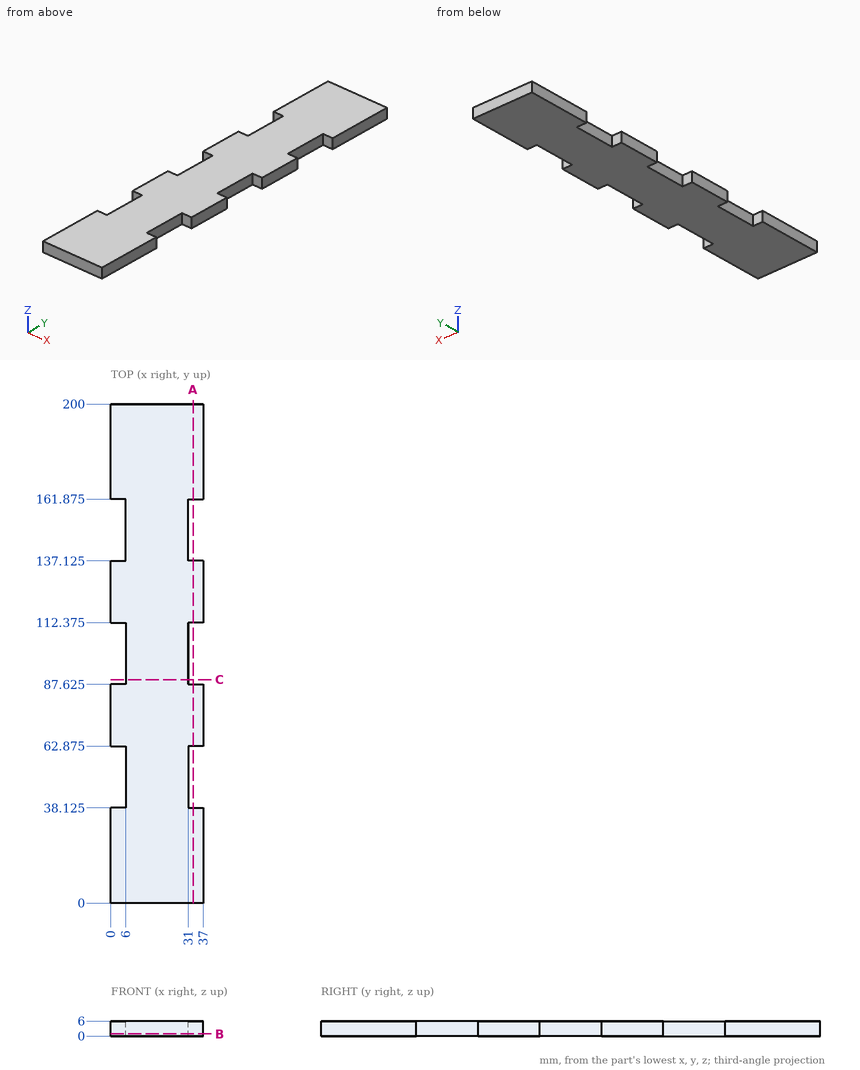
Answer from the drawing. Dimensions are ordinates in mm from the lowest x, y and z of the part. Round coordinates to 2 decimals unless told otherwise and drop trailing zeros. Loops run counter-clockwise (first coordinate to the right, second up) from the corner with the lowest first, then second, coordinate; pieces in that order, holes last.
Q1. Section C-C on y = 89.5 is taken. Write down the section's boundary in (x, z).
Q2. Each of these flat-tipped pins is pushed along its axis until it touches: pin 1 (3 mm diameter, centred on y = 148.5, z = 3, fed in from +X); pin 2 (1 mm diameter, centred on y = 49, z = 3, fed in from -X). Where does it stop, or does it pass through?
Q3. Section B-B on z = 0.9 is taken. Write down the section's boundary in (x, y) (3 decimals), and give its area (3 significant figures).
Q4. Consider probe 1 along Y at (x, z) = (5.5, 1.25) (3 decimals); probe 2 along X at (y, z) = (150.5, 3.6). Determine where each line is inside the solid, lowest interval first.
Q5. Section A-A on x = 33 is taken. Write down the section's boundary in (y, z) (3 decimals).
Output:
1. outline: (6, 0) - (31, 0) - (31, 6) - (6, 6) - close
2. pin 1: stops at x = 31
2. pin 2: stops at x = 6
3. outline: (0, 0) - (37, 0) - (37, 38.125) - (31, 38.125) - (31, 62.875) - (37, 62.875) - (37, 87.625) - (31, 87.625) - (31, 112.375) - (37, 112.375) - (37, 137.125) - (31, 137.125) - (31, 161.875) - (37, 161.875) - (37, 200) - (0, 200) - (0, 161.875) - (6, 161.875) - (6, 137.125) - (0, 137.125) - (0, 112.375) - (6, 112.375) - (6, 87.625) - (0, 87.625) - (0, 62.875) - (6, 62.875) - (6, 38.125) - (0, 38.125) - close
3. area: 6,510 mm2
4. probe 1: y = 0 to 38.125, 62.875 to 87.625, 112.375 to 137.125, 161.875 to 200
4. probe 2: x = 6 to 31
5. outline: (0, 0) - (38.125, 0) - (38.125, 6) - (0, 6) - close; (62.875, 0) - (87.625, 0) - (87.625, 6) - (62.875, 6) - close; (112.375, 0) - (137.125, 0) - (137.125, 6) - (112.375, 6) - close; (161.875, 0) - (200, 0) - (200, 6) - (161.875, 6) - close
